The figure shows three views and two pictorial views of one solid part (mm, origin at its lowest corner). Answer the questions. Round coordinates to 2 decimals unless told otherwise and drop trailing zeros. Order: outer loops, then holes, each group sorted by start corner. A loop starts at its lowest first (then second) coordinate and runs counter-clockwise, first axis right, second up. Notation, with made-up numbers: (50.25, 38) -> (65.25, 38) arc R29 cw to (65.25, 58) -> close; hole circle Ø2 at (-29, -2). An arc over 180 degrees is marked (long way). Answer as a JSON object with one key per item and string values. Group by question number.
Item 1: Section C-C, the plane z = 2.45 is taken. Write down the section's boundary in (x, y), plus the area to 3 significant figures.
Item 2: Section A-A, the plane x = 14 is taken. Write down the section's boundary in (y, z), plus the area to 3 significant figures.
Item 3: Given P1, Ø3, axis at x = 4.5, z = 4, coming from the -Y side; P2, Ø1, axis at y = 8, z = 4, coming from the +X side, each flat-ended and moving along its own axis, determine where each tip first touches the part or whether it passes through.
Item 4: The mould has two halves that part along X. Classify the marked faces 1, 2 and 3: pulls with the +X half, pulls with the -X half, needs draft (parallel to the pull), parting line crosses it, or undercut.
Item 5: Consider probe 1 along Y at (x, z) = (14, 2.3); probe 2 along Y at (x, z) = (20.75, 2.9); probe 3 along X at (y, z) = (6.5, 2.45). Determine where each line is inside the solid, lowest interval first. Write a range as from..to.
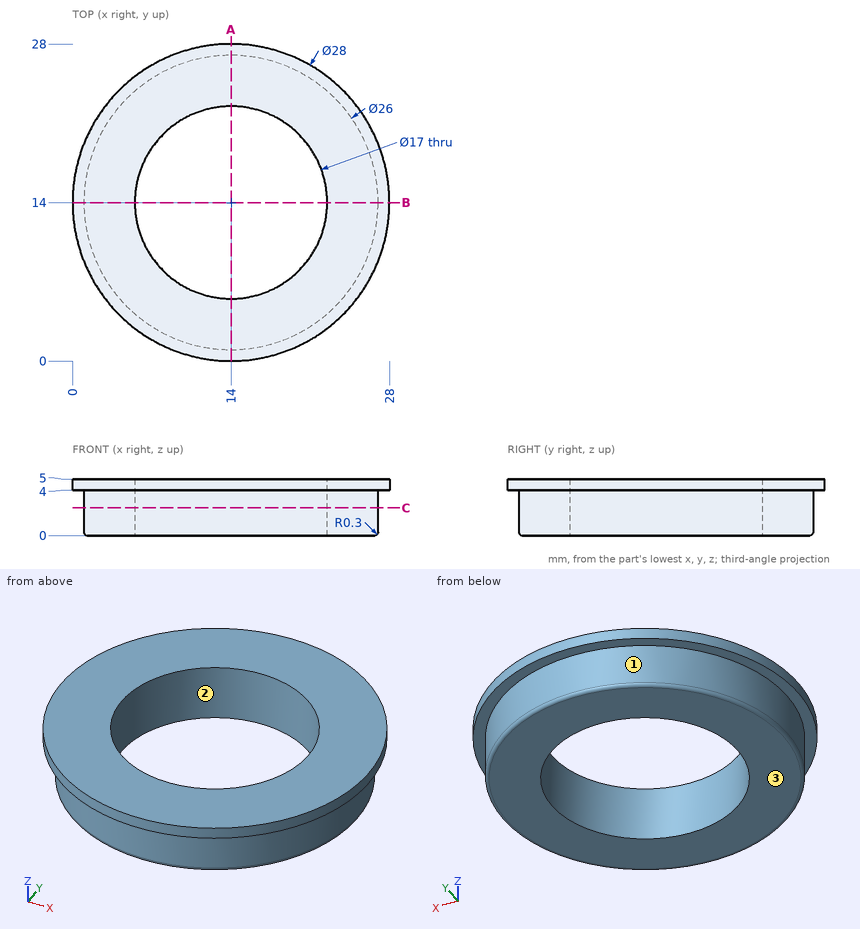
Values found:
{
 "1": {"outline": "circle Ø26 at (14, 14); hole circle Ø17 at (14, 14)", "area": "304 mm2"},
 "2": {"outline": "(0, 4) -> (1, 4) -> (1, 0.3) arc R0.3 ccw to (1.3, 0) -> (5.5, 0) -> (5.5, 5) -> (0, 5) -> close; (22.5, 0) -> (26.7, 0) arc R0.3 ccw to (27, 0.3) -> (27, 4) -> (28, 4) -> (28, 5) -> (22.5, 5) -> close", "area": "47.0 mm2"},
 "3": {"P1": "y = 2.51", "P2": "x = 26.87"},
 "4": {"face 1": "parting line crosses it", "face 2": "undercut", "face 3": "needs draft"},
 "5": {"probe 1": "1..5.5, 22.5..27", "probe 2": "2.89..8.83, 19.17..25.11", "probe 3": "3.38..10, 18..24.62"}
}
